Here's how the part is built. I have some questions about the finished solid (model axes, mm). A direction names the side the tool comes from. Give positions to 0.01 mm unless a question says otherwise; leave off trailing zeros. Loops run counter-clockwise (first coordinate to the right, second up) from the corner with the lowest first, then second, coordinate; pieces in that order, holes last. Notation, with made-up numbers: (35.25, 19.25) - (41.25, 19.25) arc R15 cw to (41.25, 39.25) - close; hole circle Ø10 at (26.5, -39.75). An arc over 180 degrees is marked (long way). One line per item, written item: value. Start each with the question number.
Autodesk Inventor part; units mm, degrees
ref_plane "YZ Plane" through (0, 0, 0) normal (1, 0, 0) x (0, 1, 0)
ref_plane "XZ Plane" through (0, 0, 0) normal (0, 1, 0) x (-1, 0, 0)
ref_plane "XY Plane" through (0, 0, 0) normal (0, 0, 1) x (1, 0, 0)
sketch "Náčrt1" plane through (0, 0, 0) normal (0, 0, 1) x (1, 0, 0)
  line L0 (0, 0) -> (11, 0)
  line L1 (11, 0) -> (11, 11)
  line L2 (11, 11) -> (0, 11)
  line L3 (0, 11) -> (0, 0)
  dimension "d0" = 11
  dimension "d1" = 11
extrude "Vysunutí1" add sketch "Náčrt1" along normal blind 3
sketch "Náčrt2" plane through (0, 0, 3) normal (0, 0, 1) x (1, 0, 0)
  circle A0 centre (5.5, 5.5) radius 3
  line L0 (0, 0) -> (11, 0)
  point P0 (5.5, 0)
  dimension "d4" = 6
  dimension "d5" = 5.5
extrude "Vysunutí2" add sketch "Náčrt2" along normal blind 8
sketch "Náčrt3" plane through (5.5, 5.5, 11) normal (0, 0, 1) x (1, 0, 0)
  circle A0 centre (0, 0) radius 0.75
  point P0 (-5.5, -5.5)
  dimension "d8" = 1.5
extrude "Vysunutí3" cut sketch "Náčrt3" against normal through all
properties part number "oparil"
(1) If we section it at D-D on y = 7: List the corners of the cut face in (x, z) for me, plus the area to 3 significant figures.
(2) For faces 5 (the face through (6, 11, 1)), 6 (the face through (8, 8, 3)), which set-ups out of +Z, -Z, +X, -X, +Y, -Y let a thin tool reach every point of the face, with its end or its side?
(3) Will this pin go through, and if not, where does the flat tip stop? pin 1 (5 mm diameter, centred on x = 1.5, z = 8, fed in from +Y).
(4) If we mould it in two halves opening along X, with no side actions, what happens to faces 1 (the face through (5.109, 2.526, 6.944)), 2 (the face through (4.75, 5.53, 5.58)), 3 (the face through (4.8, 4.9, 11)), 4 (the face through (0, 6, 1))? For each: pulls with the +X half, pulls with the -X half, needs draft (parallel to the pull), parting line crosses it, or undercut.
(5) Please list where these lines run through material, in increasing order: probe 1 along Y at (x, z) = (5.5, 8); probe 2 along Y at (x, z) = (5.5, 2.5); probe 3 along Z at (x, y) = (3, 9). Write a range as from..to.
(6) If we section it at A-A on y = 5.5: List the corners of the cut face in (x, z) for me.
(7) If we section it at C-C on z = 8: List the corners of the cut face in (x, y) for me.
Found:
1. outline: (0, 0) - (11, 0) - (11, 3) - (8.1, 3) - (8.1, 11) - (2.9, 11) - (2.9, 3) - (0, 3) - close
1. area: 74.6 mm^2
2. face 5: +Z, -Z, +X, -X, +Y
2. face 6: +Z
3. pin 1: y = 8.1
4. face 1: parting line crosses it
4. face 2: undercut
4. face 3: needs draft
4. face 4: pulls with the -X half
5. probe 1: 2.5..4.75, 6.25..8.5
5. probe 2: 0..4.75, 6.25..11
5. probe 3: 0..3
6. outline: (0, 0) - (4.75, 0) - (4.75, 11) - (2.5, 11) - (2.5, 3) - (0, 3) - close; (6.25, 0) - (11, 0) - (11, 3) - (8.5, 3) - (8.5, 11) - (6.25, 11) - close
7. outline: circle Ø6 at (5.5, 5.5); hole circle Ø1.5 at (5.5, 5.5)
